Autodesk Inventor part; units mm, degrees
ref_plane "YZ Plane" through (0, 0, 0) normal (1, 0, 0) x (0, 1, 0)
ref_plane "XZ Plane" through (0, 0, 0) normal (0, 1, 0) x (-1, 0, 0)
ref_plane "XY Plane" through (0, 0, 0) normal (0, 0, 1) x (1, 0, 0)
sketch "Sketch1" plane through (0, 0, 0) normal (0, 0, 1) x (1, 0, 0)
  line L0 (0, 0) -> (38.1, 0)
  line L1 (38.1, 0) -> (38.1, 101.6)
  line L2 (38.1, 101.6) -> (0, 101.6)
  line L3 (0, 101.6) -> (0, 0)
  dimension "d0" = 38.1
  dimension "d1" = 101.6
extrude "Extrusion1" add sketch "Sketch1" along normal blind 3
sketch "Sketch2" plane through (0, 0, 3) normal (0, 0, 1) x (1, 0, 0)
  line L0 (0, 0) -> (38.1, 0)
  line L1 (38.1, 0) -> (38.1, 101.6)
  line L2 (38.1, 101.6) -> (0, 101.6)
  line L3 (0, 101.6) -> (0, 0)
  line L4 (38.1, 12.8016) -> (35.1, 12.8016)
  line L5 (35.1, 12.8016) -> (35.1, 25.2984)
  line L6 (35.1, 25.2984) -> (38.1, 25.2984)
  line L7 (38.1, 25.2984) -> (38.1, 12.8016)
  line L8 (35.1, 38.2016) -> (35.1, 50.6984)
  line L9 (35.1, 50.6984) -> (38.1, 50.6984)
  line L10 (38.1, 38.2016) -> (35.1, 38.2016)
  line L11 (38.1, 50.6984) -> (38.1, 38.2016)
  line L12 (35.1, 63.6016) -> (35.1, 76.0984)
  line L13 (35.1, 76.0984) -> (38.1, 76.0984)
  line L14 (38.1, 63.6016) -> (35.1, 63.6016)
  line L15 (38.1, 76.0984) -> (38.1, 63.6016)
  line L16 (35.1, 89.0016) -> (35.1, 101.4984)
  line L17 (35.1, 101.4984) -> (38.1, 101.4984)
  line L18 (38.1, 89.0016) -> (35.1, 89.0016)
  line L19 (38.1, 101.4984) -> (38.1, 89.0016)
  line L20 (0, 0) -> (38.1, 0) construction
  line L21 (19.05, 0) -> (19.05, 101.6) construction
  line L22 (0, 12.8016) -> (3, 12.8016)
  line L23 (3, 12.8016) -> (3, 25.2984)
  line L24 (3, 25.2984) -> (0, 25.2984)
  line L25 (3, 38.2016) -> (3, 50.6984)
  line L26 (3, 50.6984) -> (0, 50.6984)
  line L27 (0, 38.2016) -> (3, 38.2016)
  line L28 (3, 63.6016) -> (3, 76.0984)
  line L29 (3, 76.0984) -> (0, 76.0984)
  line L30 (0, 63.6016) -> (3, 63.6016)
  line L31 (0, 76.0984) -> (0, 63.6016)
  line L32 (3, 89.0016) -> (3, 101.4984)
  line L33 (3, 101.4984) -> (0, 101.4984)
  line L34 (0, 89.0016) -> (3, 89.0016)
  line L35 (0, 101.4984) -> (0, 89.0016)
  line L36 (0, 38.2016) -> (0, 50.6984)
  line L37 (0, 101.6) -> (0, 0)
  line L38 (0, 12.8016) -> (0, 25.2984)
  dimension "d4" = 12.4968
  dimension "d5" = 12.8016
  dimension "d6" = 3
  dimension "d9" = 25.4
extrude "Extrusion2" cut sketch "Sketch2" against normal blind 3 contours L3 L24 L23 L22 | L4 L5 L6 L1 | L3 L26 L25 L27 | L10 L8 L9 L1 | L3 L29 L28 L30 | L14 L12 L13 L1 | L3 L33 L32 L34 | L18 L16 L17 L1
sketch "Sketch3" plane through (0, 0, 3) normal (0, 0, 1) x (1, 0, 0)
  line L0 (35.1, 76.0984) -> (38.1, 76.0984)
  line L1 (38.1, 76.0984) -> (38.1, 89.0016)
  line L2 (38.1, 89.0016) -> (35.1, 89.0016)
  line L3 (35.1, 89.0016) -> (35.1, 101.4984)
  line L4 (35.1, 101.4984) -> (38.1, 101.4984)
  line L5 (38.1, 101.4984) -> (38.1, 101.6)
  line L6 (38.1, 101.6) -> (0, 101.6)
  line L7 (0, 101.6) -> (0, 101.4984)
  line L8 (0, 0) -> (38.1, 0)
  line L9 (38.1, 0) -> (38.1, 12.8016)
  line L10 (38.1, 12.8016) -> (35.1, 12.8016)
  line L11 (35.1, 12.8016) -> (35.1, 25.2984)
  line L12 (35.1, 25.2984) -> (38.1, 25.2984)
  line L13 (38.1, 25.2984) -> (38.1, 38.2016)
  line L14 (38.1, 38.2016) -> (35.1, 38.2016)
  line L15 (35.1, 38.2016) -> (35.1, 50.6984)
  line L16 (35.1, 50.6984) -> (38.1, 50.6984)
  line L17 (38.1, 50.6984) -> (38.1, 63.6016)
  line L18 (38.1, 63.6016) -> (35.1, 63.6016)
  line L19 (35.1, 63.6016) -> (35.1, 76.0984)
  line L20 (38.1, 101.4984) -> (35.1, 101.4984)
  line L21 (38.1, 101.6) -> (35.1, 101.6)
  line L22 (35.1, 101.6) -> (35.1, 101.4984)
  line L23 (35.1, 101.4984) -> (38.1, 101.4984)
  line L24 (38.1, 101.4984) -> (38.1, 101.6)
  line L25 (3, 38.2016) -> (0, 38.2016)
  line L26 (0, 38.2016) -> (0, 25.2984)
  line L27 (0, 25.2984) -> (3, 25.2984)
  line L28 (3, 25.2984) -> (3, 12.8016)
  line L29 (3, 12.8016) -> (0, 12.8016)
  line L30 (0, 12.8016) -> (0, 0)
  line L31 (0, 101.4984) -> (3, 101.4984)
  line L32 (3, 101.4984) -> (3, 89.0016)
  line L33 (3, 89.0016) -> (0, 89.0016)
  line L34 (0, 89.0016) -> (0, 76.0984)
  line L35 (0, 76.0984) -> (3, 76.0984)
  line L36 (3, 76.0984) -> (3, 63.6016)
  line L37 (3, 63.6016) -> (0, 63.6016)
  line L38 (0, 63.6016) -> (0, 50.6984)
  line L39 (0, 50.6984) -> (3, 50.6984)
  line L40 (3, 50.6984) -> (3, 38.2016)
  line L41 (3, 101.4984) -> (0, 101.4984)
  line L42 (0, 101.6) -> (3, 101.6)
  line L43 (3, 101.6) -> (3, 101.4984)
  line L44 (3, 101.4984) -> (0, 101.4984)
  line L45 (0, 101.4984) -> (0, 101.6)
extrude "Extrusion3" cut sketch "Sketch3" against normal blind 3 contours L22 L6 L5 L4 | L43 L31 L7 L6
properties part number "WallBend"
Part model, mm, in its own coordinate system. A direction names the side the tool comes from. Round coordinates to 2 decimals unless told otherwise and drop trailing zeros. Write each loop counter-clockwise with the first axis right and the second up, starting at its lowest first coordinate (ties: lowest second). Pieces come first, ordered by that corner, then holes. Notation, with made-up numbers: (19, 77) -> (43, 77) arc R10 ccw to (43, 95) -> close; hole circle Ø2 at (-5.75, 29.5). An arc over 180 degrees is marked (long way). Return JSON: item names as keys, results as strings. Group by question number.
Q1. Which spindle directions (+Z, -Z, +X, -X, +Y, -Y) get a long thin tool onto all of the face, cutting with end or side? Do faces 1 (the flat face through (2, 25.298, 2)), 2 (the flat face through (37, 12.802, 2)), 3 (the flat face through (0, 6, 1)). Say none if no direction does.
Q2. Mould opens along Y. For faces 4 (the flat face through (19, 0, 1)), 5 (the flat face through (19, 52, 0)), 6 (the flat face through (1, 12.802, 2)) say: pulls with the +Y half, pulls with the -Y half, needs draft (parallel to the pull), parting line crosses it, or undercut.
Q3. Probe L1, parallel to Y at x = 2, z = 0.75; L2, parallel to X at y = 38.5, z = 0.3. List the from-to ranges inside material, lowest first. Write a range as [from, to].
Q4. Saw through at B-B on y = 46.5. Write the cut outline in (x, z).
Q5. Pin check, flat tips, straight feed: pin 1 (0.9 mm diameter, centred on x = 1.5, z = 2, fed in from +Y); pin 2 (1.5 mm diameter, centred on y = 72, z = 1, fed in from +X); pin 3 (1.5 mm diameter, centred on y = 42, z = 1.5, fed in from -X). Stop position of each tip, or through.
Answer:
{
 "1": {"face 1": "+Z, -Z, -X", "face 2": "+Z, -Z, +X", "face 3": "+Z, -Z, -X, +Y, -Y"},
 "2": {"face 4": "pulls with the -Y half", "face 5": "needs draft", "face 6": "undercut"},
 "3": {"L1": "[0, 12.8], [25.3, 38.2], [50.7, 63.6], [76.1, 89]", "L2": "[3, 35.1]"},
 "4": {"outline": "(3, 0) -> (35.1, 0) -> (35.1, 3) -> (3, 3) -> close"},
 "5": {"pin 1": "y = 89", "pin 2": "x = 35.1", "pin 3": "x = 3"}
}
